from build123d import *

# Parameters (mm, degrees)
F1_DEPTH = 20
F2_DEPTH = 15
F3_R     = 5
F4_DEPTH = 20.001
F6_DEPTH = 10
F7_DEPTH = 10


with BuildPart() as f1:
    # F0 (on Front) → F1 (new body)
    with BuildSketch(Plane.XZ):
        with BuildLine():
            ThreePointArc((0, -10), (7.0710678119, -7.0710678119), (10, 0))
            ThreePointArc((10, 0), (7.0710678119, 7.0710678119), (0, 10))
            ThreePointArc((0, 10), (-10, 0), (0, -10))
        make_face()
    extrude(amount=F1_DEPTH)

    # F0 (on Front) → F2 (join)
    with BuildSketch(Plane.XZ):
        with BuildLine():
            ThreePointArc((0, 10), (7.0710678119, 7.0710678119), (10, 0))
            ThreePointArc((10, 0), (7.0710678119, -7.0710678119), (0, -10))
            Line((0, -10), (15, -10))
            Line((15, -10), (18.6824316361, -5))
            Line((18.6824316361, -5), (18.6824316361, 5))
            Line((18.6824316361, 5), (15, 10))
            Line((15, 10), (0, 10))
        make_face()
    extrude(amount=F2_DEPTH)

    # F3 (on face) → F4 (cut, through all)
    with BuildSketch(Plane.XZ.offset(20)):
        Circle(F3_R)
    extrude(amount=-F4_DEPTH, mode=Mode.SUBTRACT)

    # F5 (on face) → F6 (cut)
    with BuildSketch(Plane.XZ.offset(20)):
        with BuildLine():
            ThreePointArc((10, 0), (9.9202969627, 1.2600429248), (9.6824583655, 2.5))
            Line((9.6824583655, 2.5), (4.3301270189, 2.5))
            ThreePointArc((4.3301270189, 2.5), (4.8296291314, 1.2940952255), (5, 0))
            ThreePointArc((5, 0), (4.8296291314, -1.2940952255), (4.3301270189, -2.5))
            Line((4.3301270189, -2.5), (9.6824583655, -2.5))
            ThreePointArc((9.6824583655, -2.5), (9.9202969627, -1.2600429248), (10, 0))
        make_face()
        with BuildLine():
            Line((-4.3301270189, 2.5), (-9.6824583655, 2.5))
            ThreePointArc((-9.6824583655, 2.5), (-10, 0), (-9.6824583655, -2.5))
            Line((-9.6824583655, -2.5), (-4.3301270189, -2.5))
            ThreePointArc((-4.3301270189, -2.5), (-5, 0), (-4.3301270189, 2.5))
        make_face()
    extrude(amount=-F6_DEPTH, mode=Mode.SUBTRACT)

    # F5 (on face) → F7 (cut)
    with BuildSketch(Plane.XZ.offset(20)):
        with BuildLine():
            Line((18.6824316361, -2.5), (18.6824316361, 2.5))
            Line((18.6824316361, 2.5), (9.6824583655, 2.5))
            ThreePointArc((9.6824583655, 2.5), (9.9202969627, 1.2600429248), (10, 0))
            ThreePointArc((10, 0), (9.9202969627, -1.2600429248), (9.6824583655, -2.5))
            Line((9.6824583655, -2.5), (18.6824316361, -2.5))
        make_face()
    extrude(amount=-F7_DEPTH, mode=Mode.SUBTRACT)


solid = f1.part
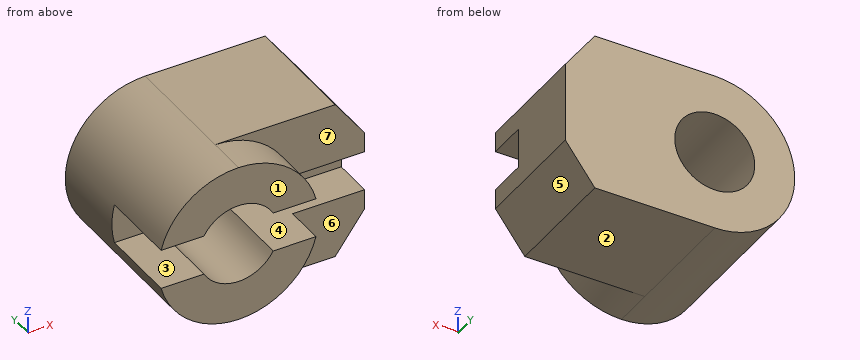
Work out the finished part from the listing and answer in its coordinate system (mm). Face numbers are marked on the shaded views. A direction names the side the tool comes from. Give positions to 0.01 mm unless a question says otherwise; leave off trailing zeros. Loops run counter-clockwise (first coordinate to the right, second up) from the corner with the lowest first, then second, coordinate; pieces in that order, holes last. Notation, with made-up numbers: (18, -9.75) -> (44, -9.75) arc R21 ccw to (44, 21.25) -> close; hole circle Ø5 at (27, 43.5). An arc over 180 degrees is marked (long way). Use a Markdown table: item, result. Add a question column.
1) The part is cut by section A-A, the plane z = 0. Determine the outline of the cut face in (x, y), plus the area to 3 significant figures.
2) Each of these flat-tipped pins is pushed along its axis until it touches: P1, Ø2.5, axis at x = -7, y = -16.5, coming from the -Z side; P2, Ø8, axis at x = 10.5, z = -5, coming from the -Y side; P3, Ø5, axis at x = -5, y = -18, coming from the -Z side; P4, Ø1.5, axis at x = 8.5, z = 1, coming from the -Y side. Where does it stop, or does it pass through?
3) For a pull along Z with two mould halves and no side action, classify the marked faces 1, 2 and 3 as +Z half, -Z half, draft (parallel to the pull), parting line (faces both ways), or undercut.
4) The part is cut by section B-B, the plane x = 13.75. Determine the outline of the cut face in (y, z).
5) The part is cut by section D-D, the plane x = 1.25. Determine the outline of the cut face in (y, z).
6) Which of the six approach directions +Z, -Z, +X, -X, +Y, -Y give full straight-line access (tool end or side, diameter ignored) to the marked faces 4, 5, 6 and 7?
7) The part is cut by section C-C, the plane y = -6.25. Determine the outline of the cut face in (x, z), plus the area to 3 significant figures.
8) Consider line 1 along Z through (x, y) = (0, -6.5); line 2 along X through (y, z) = (-6.75, 0); line 3 along Z through (x, y) = (10.5, -12.75). Determine where each line is inside the solid, lowest interval first.
Reported:
| question | item | result |
|---|---|---|
| 1 | outline | (-10, -10) -> (-5, -10) -> (-5, 0) -> (-10, 0) -> close; (5, -10) -> (18.68, -10) -> (18.68, 0) -> (5, 0) -> close |
| 1 | area | 187 mm^2 |
| 2 | P1 | stops at z = -8.18 |
| 2 | P2 | stops at y = -20 |
| 2 | P3 | stops at z = -9.68 |
| 2 | P4 | stops at y = -10 |
| 3 | face 1 | draft |
| 3 | face 2 | -Z half |
| 3 | face 3 | undercut |
| 4 | outline | (-15, -10) -> (0, -10) -> (0, 10) -> (-15, 10) -> (-15, 2.5) -> (-10, 2.5) -> (-10, -2.5) -> (-15, -2.5) -> close |
| 5 | outline | (-20, -9.92) -> (-15, -9.92) -> (-15, -10) -> (0, -10) -> (0, -4.84) -> (-20, -4.84) -> close; (-20, 4.84) -> (0, 4.84) -> (0, 10) -> (-15, 10) -> (-15, 9.92) -> (-20, 9.92) -> close |
| 6 | face 4 | +X, -X, -Y |
| 6 | face 5 | -Z, +X, +Y, -Y |
| 6 | face 6 | -Z, +X, -Y |
| 6 | face 7 | +Z, +X, -Y |
| 7 | outline | (0, -10) -> (15, -10) -> (18.68, -5) -> (18.68, 5) -> (15, 10) -> (0, 10) arc R10 ccw to start; hole circle Ø10 at (0, 0) |
| 7 | area | 434 mm^2 |
| 8 | line 1 | z = -10 to -5, 5 to 10 |
| 8 | line 2 | x = -10 to -5, 5 to 18.68 |
| 8 | line 3 | z = -10 to -2.5, 2.5 to 10 |
